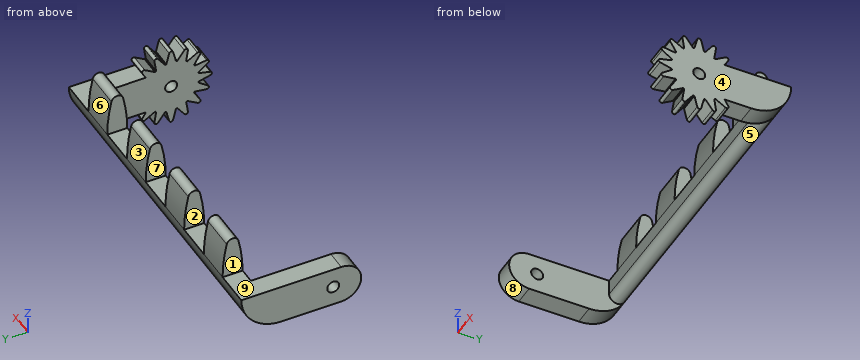
from build123d import *

# Parameters (mm, degrees)
BOSS_EXTRU_1_DEPTH               = 10
BOSS_EXTRU_2_START               = -9
BOSS_EXTRU_2_DEPTH               = 9
CONG_1_R                         = 1.5
R_P_TITION_LIN_AIRE1_COUNT       = 4
R_P_TITION_LIN_AIRE1_PITCH       = 18.5
CONG_1_OF_R_P_TITION_LIN_AIRE1_R = 1.5
ENL_V_MAT_EXTRU_1_DEPTH          = 82.974649073
ENL_V_MAT_EXTRU_1_DEPTH_BACK     = 82.974649073
ESQUISSE4_R                      = 1.5
CONG_2_RADIUS                    = 5
CONG_2_LENGTH                    = 5
CONG_3_RADIUS                    = 5
CONG_3_LENGTH                    = 5
CONG_4_R                         = 10
BOSS_EXTRU_3_START               = 73
ESQUISSE5_R                      = 1.5
BOSS_EXTRU_3_DEPTH               = 5
CONG_7_R                         = 2


with BuildPart() as part:
    # Esquisse1 → Boss.-Extru.1 (new body)
    with BuildSketch(Plane.XY):
        Polygon((-36.5, 10), (36.5, 10), (36.5, -10), (36.5, -15), (41.5, -15), (41.5, 15), (-41.5, 15), (-41.5, -15), (-36.5, -15), (-36.5, -10), align=None)
    extrude(amount=BOSS_EXTRU_1_DEPTH)

    # Esquisse2 → Boss.-Extru.2 (add)
    with BuildSketch(Plane.ZY.offset(41.5).offset(BOSS_EXTRU_2_START)):
        with BuildLine():
            Line((10, 10), (10, 15))
            ThreePointArc((10, 15), (17.110731327, 14.370095429), (24, 12.5))
            ThreePointArc((24, 12.5), (17.110731327, 10.629904571), (10, 10))
        make_face()
    boss_extru_2 = extrude(amount=-BOSS_EXTRU_2_DEPTH)

    # Congé1
    cong_1_edges = [part.edges().sort_by_distance(p)[0] for p in [
        (-28, 12.5, 24),
    ]]
    fillet(cong_1_edges, radius=CONG_1_R)

    # Répétition linéaire1: Boss.-Extru.2 ×4
    with Locations(*[(i * R_P_TITION_LIN_AIRE1_PITCH, 0, 0) for i in range(1, R_P_TITION_LIN_AIRE1_COUNT)]):
        add(boss_extru_2)

    # Congé1 of Répétition linéaire1
    cong_1_of_r_p_tition_lin_aire1_edges = [part.edges().sort_by_distance(p)[0] for p in [
        (-9.5, 12.5, 24),
        (9, 12.5, 24),
        (27.5, 12.5, 24),
    ]]
    fillet(cong_1_of_r_p_tition_lin_aire1_edges, radius=CONG_1_OF_R_P_TITION_LIN_AIRE1_R)

    # Esquisse4 → Enlèv. mat.-Extru.1 (cut, two sides: drawn at the far end of the back side and taken through both)
    with BuildSketch(Plane(origin=(-36.5, 0, 0), x_dir=(0, 0, -1), z_dir=(1, 0, 0)).offset(-ENL_V_MAT_EXTRU_1_DEPTH_BACK)):
        with Locations((-5, -8)):
            Circle(ESQUISSE4_R)
    extrude(amount=ENL_V_MAT_EXTRU_1_DEPTH + ENL_V_MAT_EXTRU_1_DEPTH_BACK, mode=Mode.SUBTRACT)

    # Congé2: full round fillet: the end face becomes a half cylinder, R = half its width
    cong_2_face = Plane((-39, -15, 5), x_dir=(1, 0, 0), z_dir=(0, -1, 0))  # on the end face: x along it, z out of the body
    cong_2_slab = cong_2_face.offset(-CONG_2_RADIUS / 2) * Box(CONG_2_LENGTH, 2 * CONG_2_RADIUS, CONG_2_RADIUS, mode=Mode.PRIVATE)  # the body's end, R deep
    cong_2_round = Plane((-39, -10, 5), x_dir=(0, -1, 0), z_dir=(1, 0, 0)) * Cylinder(CONG_2_RADIUS, CONG_2_LENGTH, mode=Mode.PRIVATE)  # its axis R under the face
    add(cong_2_slab - cong_2_round, mode=Mode.SUBTRACT)

    # Congé3: full round fillet: the end face becomes a half cylinder, R = half its width
    cong_3_face = Plane((39, -15, 5), x_dir=(1, 0, 0), z_dir=(0, -1, 0))  # on the end face: x along it, z out of the body
    cong_3_slab = cong_3_face.offset(-CONG_3_RADIUS / 2) * Box(CONG_3_LENGTH, 2 * CONG_3_RADIUS, CONG_3_RADIUS, mode=Mode.PRIVATE)  # the body's end, R deep
    cong_3_round = Plane((39, -10, 5), x_dir=(0, -1, 0), z_dir=(1, 0, 0)) * Cylinder(CONG_3_RADIUS, CONG_3_LENGTH, mode=Mode.PRIVATE)  # its axis R under the face
    add(cong_3_slab - cong_3_round, mode=Mode.SUBTRACT)

    # Congé4
    # the kernel refuses this fillet: 10 mm, written as the material it takes off along each edge
    with BuildSketch(Plane(origin=(66.5, 15, 0), x_dir=(0, -1, 0), z_dir=(-1, 0, 0))) as cong_4_piece_1:
        with BuildLine():
            CenterArc((CONG_4_R, CONG_4_R), CONG_4_R, 180, 90)
            Line((0, CONG_4_R), (0, 0))
            Line((0, 0), (CONG_4_R, 0))
        make_face()
    extrude(amount=133, mode=Mode.SUBTRACT)

    # Esquisse5 → Boss.-Extru.3 (add)
    with BuildSketch(Plane(origin=(-36.5, 0, 0), x_dir=(0, 0, -1), z_dir=(1, 0, 0)).offset(BOSS_EXTRU_3_START)):
        with BuildLine():
            Line((-14.800353701, -8.485147863), (-11.894696869, -9.209609478))
            ThreePointArc((-11.894696869, -9.209609478), (-11.865496963, -9.365632254), (-11.832766827, -9.520952824))
            Line((-11.832766827, -9.520952824), (-14.240004245, -11.302214812))
            ThreePointArc((-14.240004245, -11.302214812), (-14.404532618, -11.895484958), (-13.868688146, -12.198651174))
            Line((-13.868688146, -12.198651174), (-10.906971813, -11.756019702))
            ThreePointArc((-10.906971813, -11.756019702), (-10.820287286, -11.888991631), (-10.730609975, -12.019963846))
            Line((-10.730609975, -12.019963846), (-12.272947904, -14.586845216))
            ThreePointArc((-12.272947904, -14.586845216), (-12.197917644, -15.197917644), (-11.586845216, -15.272947904))
            Line((-11.586845216, -15.272947904), (-9.019963846, -13.730609975))
            ThreePointArc((-9.019963846, -13.730609975), (-8.888991631, -13.820287286), (-8.756019702, -13.906971813))
            Line((-8.756019702, -13.906971813), (-9.198651174, -16.868688146))
            ThreePointArc((-9.198651174, -16.868688146), (-8.895484958, -17.404532618), (-8.302214812, -17.240004245))
            Line((-8.302214812, -17.240004245), (-6.520952824, -14.832766827))
            ThreePointArc((-6.520952824, -14.832766827), (-6.365632254, -14.865496963), (-6.209609478, -14.894696869))
            Line((-6.209609478, -14.894696869), (-5.485147863, -17.800353701))
            ThreePointArc((-5.485147863, -17.800353701), (-5, -18.179392753), (-4.514852137, -17.800353701))
            Line((-4.514852137, -17.800353701), (-3.790390522, -14.894696869))
            ThreePointArc((-3.790390522, -14.894696869), (-3.634367746, -14.865496963), (-3.479047176, -14.832766827))
            Line((-3.479047176, -14.832766827), (-1.697785188, -17.240004245))
            ThreePointArc((-1.697785188, -17.240004245), (-1.104515042, -17.404532618), (-0.801348826, -16.868688146))
            Line((-0.801348826, -16.868688146), (-1.243980298, -13.906971813))
            ThreePointArc((-1.243980298, -13.906971813), (-1.111008369, -13.820287286), (-0.980036154, -13.730609975))
            Line((-0.980036154, -13.730609975), (1.586845216, -15.272947904))
            ThreePointArc((1.586845216, -15.272947904), (2.197917644, -15.197917644), (2.272947904, -14.586845216))
            Line((2.272947904, -14.586845216), (0.730609975, -12.019963846))
            ThreePointArc((0.730609975, -12.019963846), (0.820287286, -11.888991631), (0.906971813, -11.756019702))
            Line((0.906971813, -11.756019702), (3.868688146, -12.198651174))
            ThreePointArc((3.868688146, -12.198651174), (4.404532618, -11.895484958), (4.240004245, -11.302214812))
            Line((4.240004245, -11.302214812), (1.832766827, -9.520952824))
            ThreePointArc((1.832766827, -9.520952824), (1.865496963, -9.365632254), (1.894696869, -9.209609478))
            Line((1.894696869, -9.209609478), (4.800353701, -8.485147863))
            ThreePointArc((4.800353701, -8.485147863), (5.179392753, -8), (4.800353701, -7.514852137))
            Line((4.800353701, -7.514852137), (1.894696869, -6.790390522))
            ThreePointArc((1.894696869, -6.790390522), (1.865496963, -6.634367746), (1.832766827, -6.479047176))
            Line((1.832766827, -6.479047176), (4.240004245, -4.697785188))
            ThreePointArc((4.240004245, -4.697785188), (4.404532618, -4.104515042), (3.868688146, -3.801348826))
            Line((3.868688146, -3.801348826), (0.906971813, -4.243980298))
            ThreePointArc((0.906971813, -4.243980298), (0.820287286, -4.111008369), (0.730609975, -3.980036154))
            Line((0.730609975, -3.980036154), (2.272947904, -1.413154784))
            ThreePointArc((2.272947904, -1.413154784), (2.197917644, -0.802082356), (1.586845216, -0.727052096))
            Line((1.586845216, -0.727052096), (-0.980036154, -2.269390025))
            ThreePointArc((-0.980036154, -2.269390025), (-1.111008369, -2.179712714), (-1.243980298, -2.093028187))
            Line((-1.243980298, -2.093028187), (-0.801348826, 0.868688146))
            ThreePointArc((-0.801348826, 0.868688146), (-1.104515042, 1.404532618), (-1.697785188, 1.240004245))
            Line((-1.697785188, 1.240004245), (-3.479047176, -1.167233173))
            ThreePointArc((-3.479047176, -1.167233173), (-3.634367746, -1.134503037), (-3.790390522, -1.105303131))
            Line((-3.790390522, -1.105303131), (-4.514852137, 1.800353701))
            ThreePointArc((-4.514852137, 1.800353701), (-5, 2.179392753), (-5.485147863, 1.800353701))
            Line((-5.485147863, 1.800353701), (-6.209609478, -1.105303131))
            ThreePointArc((-6.209609478, -1.105303131), (-6.365632254, -1.134503037), (-6.520952824, -1.167233173))
            Line((-6.520952824, -1.167233173), (-8.302214812, 1.240004245))
            ThreePointArc((-8.302214812, 1.240004245), (-8.895484958, 1.404532618), (-9.198651174, 0.868688146))
            Line((-9.198651174, 0.868688146), (-8.756019702, -2.093028187))
            ThreePointArc((-8.756019702, -2.093028187), (-8.888991631, -2.179712714), (-9.019963846, -2.269390025))
            Line((-9.019963846, -2.269390025), (-11.586845216, -0.727052096))
            ThreePointArc((-11.586845216, -0.727052096), (-12.197917644, -0.802082356), (-12.272947904, -1.413154784))
            Line((-12.272947904, -1.413154784), (-10.730609975, -3.980036154))
            ThreePointArc((-10.730609975, -3.980036154), (-10.820287286, -4.111008369), (-10.906971813, -4.243980298))
            Line((-10.906971813, -4.243980298), (-13.868688146, -3.801348826))
            ThreePointArc((-13.868688146, -3.801348826), (-14.404532618, -4.104515042), (-14.240004245, -4.697785188))
            Line((-14.240004245, -4.697785188), (-11.832766827, -6.479047176))
            ThreePointArc((-11.832766827, -6.479047176), (-11.865496963, -6.634367746), (-11.894696869, -6.790390522))
            Line((-11.894696869, -6.790390522), (-14.800353701, -7.514852137))
            ThreePointArc((-14.800353701, -7.514852137), (-15.179392753, -8), (-14.800353701, -8.485147863))
        make_face()
        with Locations((-5, -8)):
            Circle(ESQUISSE5_R, mode=Mode.SUBTRACT)
    extrude(amount=BOSS_EXTRU_3_DEPTH)

    # Congé7
    cong_7_edges = [part.edges().sort_by_distance(p)[0] for p in [
        (0, 10, 1.339745962),
    ]]
    fillet(cong_7_edges, radius=CONG_7_R)


solid = part.part
Geometry: final body of the model. Coordinates: model frame, mm. Face numbers are marked on the shaded views. A direction names the side the tool comes from. Round coordinates to 2 decimals unless told otherwise and drop trailing zeros. Order: outer loops, then holes, each group sorted by start corner. A loop starts at its lowest first (then second) coordinate and runs counter-clockwise, first axis right, second up.
Q1. Access query for the marked faces 5, 6, 7, 8 and 9. Directions: +Z, -Z, +X, -X, +Y, -Y. A direction counts if a zero-diameter tool reaches every point of the face in a straight line with its end or side. Return the directions, or none.
Result sheet:
face 5: -Z
face 6: +Z, +X, -X, +Y
face 7: +Z, +Y, -Y
face 8: -X, -Y
face 9: +Z, -X, +Y, -Y
Q2. Mould query, pull axis X, two halves, no side actions, for the marked faces 1, 2, 3 and 4. Classes: released by +X, released by -X, zero draft, split by the parting line, or undercut.
Result sheet:
face 1: released by -X
face 2: undercut
face 3: zero draft
face 4: released by +X
Q3. Section A-A, the plane x = -2.5. Output: boundary loops of the cut face in (y, z), and give its area (3 significant figures).
Result sheet:
outline: (10, 6.13) arc R2 ccw to (13.75, 5.16) arc R10 ccw to (15, 10) - (10, 10) - close
area: 24.7 mm2
Q4. Material intervals for probe 1 along X at (y, z) = (-12.5, 2.75); probe 2 along Z at (x, y) = (40, -8); probe 3 along Z at (x, y) = (-38.3, -8), sorted ascending.
Result sheet:
probe 1: x = -41.5 to -36.5, 36.5 to 41.5
probe 2: z = -5.18 to 3.5, 6.5 to 15.18
probe 3: z = 0 to 3.5, 6.5 to 10
Q5. Pin query (flat end, axial travel): pin 1 (6 mm diameter, centred on x = -21, z = 1, fed in from -Y); pin 2 (2.5 mm diameter, centred on y = 11.5, z = 17, fed in from +X); pin 3 (2.5 mm diameter, centred on x = 18.5, y = 13.5, fed in from +Z); pin 4 (5.5 mm diameter, centred on x = -40, y = -5.5, fed in from -Z). Return the tip coordinate at first contact, or that it passes through.
Result sheet:
pin 1: passes through
pin 2: stops at x = 32
pin 3: stops at z = 10
pin 4: stops at z = 0
